Read the model definition and answer for the solid it produces. Units are mm, in the model's axes. A direction names the side the tool comes from. Round coordinates to 2 decimals unless told otherwise and drop trailing zeros. Write each loop counter-clockwise with the first axis right and the second up, starting at its lowest first coordinate (ties: lowest second). Pieces come first, ordered by that corner, then holes. Notation, with made-up numbers: (2.5, 65) -> (32.5, 65) arc R10 cw to (32.5, 71) -> close; hole circle Ø5 at (34.25, 14.25). An arc over 180 degrees is marked (long way). Return JSON: item names as keys, results as strings. Group by question number.
(1) A cutting plane is placed at D-D on y = 19.25. Give the vertices of the cut face in (x, z).
(2) A cutting plane is placed at A-A on y = 11. Give the vertices of the cut face in (x, z).
(3) Straight lines are drawn through the part: line 1 (X direction, y = 13.75, z = -7); line 2 (X direction, y = 7.5, z = -24); line 3 (Z direction, x = -27, y = 10). For each, find the intervals that lie inside material, in ascending order.
(4) Given pin 1 (12 mm diameter, centred on y = 7.5, z = -21.5, fed in from +X); pin 2 (6 mm diameter, centred on x = 11, y = 5.5, fed in from +Z); pin 3 (1.3 mm diameter, centred on y = 9, z = -59.5, fed in from -X), each flat-ended and moving along its own axis, determine where each tip first touches the part or whether it passes through.
(5) A cutting plane is placed at C-C on x = -31.5. Give the vertices of the cut face in (y, z), then the cut area to 3 significant figures.
(6) A cutting plane is placed at B-B on z = -11.7. Give the vertices of the cut face in (x, y).
(7) The mould has two halves that part along Y. Classify faces 1 (the cylindrical face through (8.87, 5.37, -44)), 2 (the flat face through (0, 11, -60)), 3 (the flat face through (-15, 22, -30)): released by +Y, released by -Y, zero draft, split by the parting line, or undercut.
(8) For faces 4 (the flat face through (-15, 0, -30)), 5 (the flat face through (-15, 11, -59)), 6 (the cylindrical face through (-33.437, 2.128, -7.086)), determine the directions among +Z, -Z, +X, -X, +Y, -Y from which every point of the face is accessible in a straight line to the end or side of a thin tool.
```python
from build123d import *

# Parameters (mm, degrees)
SKETCH1_W           = 29
SKETCH1_H           = 59
BOSS_EXTRUDE1_DEPTH = 22
SKETCH4_R           = 9.25
BOSS_EXTRUDE4_DEPTH = 18
SKETCH5_R           = 10
BOSS_EXTRUDE5_DEPTH = 9


with BuildPart() as part:
    # Sketch1 → Boss-Extrude1 (new body)
    with BuildSketch(Plane(origin=(0, 0, 0), x_dir=(1, 0, 0), z_dir=(0, 1, 0))):
        with Locations((-14.5, 29.5)):
            Rectangle(SKETCH1_W, SKETCH1_H)
    extrude(amount=BOSS_EXTRUDE1_DEPTH)

    # Sketch4 → Boss-Extrude4 (add)
    with BuildSketch(Plane(origin=(0, 0, 0), x_dir=(0, 0, -1), z_dir=(1, 0, 0))):
        with Locations((51.3375, 11)):
            Circle(SKETCH4_R)
    extrude(amount=BOSS_EXTRUDE4_DEPTH)

    # Sketch5 → Boss-Extrude5 (add)
    with BuildSketch(Plane.ZY.offset(29)):
        with Locations((-11.7, 11)):
            Circle(SKETCH5_R)
    extrude(amount=BOSS_EXTRUDE5_DEPTH)


solid = part.part
```
Checks:
{
 "1": {"outline": "(-38, -17.35) -> (-29, -17.35) -> (-29, -59) -> (0, -59) -> (0, -55.52) -> (18, -55.52) -> (18, -47.15) -> (0, -47.15) -> (0, 0) -> (-29, 0) -> (-29, -6.05) -> (-38, -6.05) -> close"},
 "2": {"outline": "(-38, -21.7) -> (-29, -21.7) -> (-29, -59) -> (0, -59) -> (0, -60.59) -> (18, -60.59) -> (18, -42.09) -> (0, -42.09) -> (0, 0) -> (-29, 0) -> (-29, -1.7) -> (-38, -1.7) -> close"},
 "3": {"line 1": "x = -38 to 0", "line 2": "x = -29 to 0", "line 3": "z = -59 to 0"},
 "4": {"pin 1": "stops at x = 0", "pin 2": "stops at z = -42.43", "pin 3": "stops at x = -29"},
 "5": {"outline": "circle Ø20 at (11, -11.7)", "area": "314 mm^2"},
 "6": {"outline": "(-38, 1) -> (-29, 1) -> (-29, 0) -> (0, 0) -> (0, 22) -> (-29, 22) -> (-29, 21) -> (-38, 21) -> close"},
 "7": {"face 1": "split by the parting line", "face 2": "zero draft", "face 3": "released by +Y"},
 "8": {"face 4": "+Z, -Z, +X, -X, -Y", "face 5": "-Z, -X, +Y, -Y", "face 6": "-X"}
}
